Geometry: final body of the model. Coordinates: model frame, mm. A direction names the side the tool comes from. Give positions to 0.01 mm unless a question says otherwise; leave off trailing zeros. Write each loop counter-clockwise with the first axis right and the second up, starting at its lowest first coordinate (ties: lowest second). Pieces come first, ordered by that corner, then holes. Notation, with made-up numbers: M 4,58.25 L 48,58.25 A4 ccw 48,62.25 Z; hole C 33,24.5 d7. An arc over 180 degrees is marked long. Use one line per item in the form item = value. Start each with the question number.
Item 1: Section query A-A on z = -1.5. Return loops of the section in (x, y), then the cut area to 3 significant figures.
Item 2: Access query for faces 1 (the flat face through (-7.9, 2, 5)), 2 (the flat face through (-12.5, 0, 2)), 3 (the flat face through (10.25, -4, 11)), 4 (the flat face through (14.25, -4, 9)). Directions: +Z, -Z, +X, -X, +Y, -Y. A direction counts if a zero-diameter tool reaches every point of the face in a straight line with its end or side. Return the directions, or none.
Item 3: Material intervals for line 1 along Z through (x, y) = (21.3, 0); line 2 along Z through (x, y) = (12.25, -4.2); line 3 along X through (y, z) = (-3, 2), sorted ascending. Write a range as from..to.
Item 4: Contact query for flat-ended pins moving along their axis: P1, Ø2, axis at y = 3, z = 3, coming from the -X side; P2, Ø1.3, axis at y = -3.5, z = 11, coming from the +X side; P3, Ø6, axis at x = 16.5, z = 8.5, coming from the +Y side. Output: stop coordinate, or through.
Item 5: Section query B-B on x = 17.5. Return loops of the section in (y, z).
Item 6: Section query D-D on y = -1.75. Return loops of the section in (x, z), then the cut area to 3 significant figures.
Item 7: Section query C-C on z = 14.9. Return loops of the section in (x, y), then the cut area to 3 significant figures.
Item 8: Pull-direction query (X, two-part tool) for faces 5 (the flat face through (-12, -4, 16.9)), 6 (the cylindrical face through (-16.576, -0.383, 0.71)), 7 (the flat face through (-14.25, -4, 9)); classes: released by +X, released by -X, zero draft, split by the parting line, or undercut.
from build123d import *

# Parameters (mm, degrees)
F1_DEPTH = 4.5
F2_R     = 0.75
F3_DEPTH = 43.801
F4_R     = 1
F5_DEPTH = 1.2
F6_R     = 1
F6_W     = 15.8
F6_H     = 4.5
F7_DEPTH = 11.401


with BuildPart() as f1:
    # F0 (on Front) → F1 (new body, symmetric)
    with BuildSketch(Plane.XZ):
        Polygon((12.5, 4), (12.5, 0), (20.5, 0), (20.5, -6), (21.9, -6), (21.9, 1.4), (13.9, 1.4), (13.9, 5.4), (-13.9, 5.4), (-13.9, 1.4), (-21.9, 1.4), (-21.9, -6), (-20.5, -6), (-20.5, 0), (-12.5, 0), (-12.5, 4), align=None)
    extrude(amount=F1_DEPTH, both=True)

    # F2 (on face) → F3 (cut, through all)
    with BuildSketch(Plane.YZ.offset(21.9)):
        with Locations((0, -3.5)):
            Circle(F2_R)
    extrude(amount=-F3_DEPTH, mode=Mode.SUBTRACT)

    # F4 (on face) → F5 (join)
    with BuildSketch(Plane.XZ.offset(4.5)):
        Polygon((14.25, 16.9), (10.25, 16.9), (10.25, 5.4), (13.9, 5.4), (13.9, 1.4), (14.25, 1.4), align=None)
        with Locations((12.25, 14.9)):
            Circle(F4_R, mode=Mode.SUBTRACT)
        Polygon((-10.25, 16.9), (-14.25, 16.9), (-14.25, 1.4), (-13.9, 1.4), (-13.9, 5.4), (-10.25, 5.4), align=None)
        with Locations((-12.25, 14.9)):
            Circle(F4_R, mode=Mode.SUBTRACT)
    extrude(amount=-F5_DEPTH)

    # F6 (on face) → F7 (cut, through all)
    with BuildSketch(Plane.XY.offset(5.4)):
        with Locations((-17.5, 0)):
            Circle(F6_R)
        with Locations((17.5, 0)):
            Circle(F6_R)
        with Locations((0, 2.25)):
            Rectangle(F6_W, F6_H)
    extrude(amount=-F7_DEPTH, mode=Mode.SUBTRACT)


solid = f1.part
Answer sheet:
q1.outline = M -21.9,-4.5 L -20.5,-4.5 L -20.5,4.5 L -21.9,4.5 Z; M 20.5,-4.5 L 21.9,-4.5 L 21.9,4.5 L 20.5,4.5 Z
q1.area = 25.2 mm2
q2.face_1 = +Z, -Z, +Y
q2.face_2 = -Z, +Y, -Y
q2.face_3 = +Z, +Y, -Y
q2.face_4 = +Z, +X, +Y, -Y
q3.line_1 = -6..-4.25, -2.75..1.4
q3.line_2 = 4..13.9, 15.9..16.9
q3.line_3 = -13.9..-12.5, 12.5..13.9
q4.P1 = -13.9
q4.P2 = 14.25
q4.P3 = -3.3
q5.outline = M -4.5,0 L -1,0 L -1,1.4 L -4.5,1.4 Z; M 1,0 L 4.5,0 L 4.5,1.4 L 1,1.4 Z
q6.outline = M -21.9,-6 L -20.5,-6 L -20.5,0 L -12.5,0 L -12.5,4 L 12.5,4 L 12.5,0 L 20.5,0 L 20.5,-6 L 21.9,-6 L 21.9,1.4 L 13.9,1.4 L 13.9,5.4 L -13.9,5.4 L -13.9,1.4 L -21.9,1.4 Z
q6.area = 89.3 mm2
q7.outline = M -14.25,-4.5 L -13.25,-4.5 L -13.25,-3.3 L -14.25,-3.3 Z; M -11.25,-4.5 L -10.25,-4.5 L -10.25,-3.3 L -11.25,-3.3 Z; M 10.25,-4.5 L 11.25,-4.5 L 11.25,-3.3 L 10.25,-3.3 Z; M 13.25,-4.5 L 14.25,-4.5 L 14.25,-3.3 L 13.25,-3.3 Z
q7.area = 4.80 mm2
q8.face_5 = zero draft
q8.face_6 = undercut
q8.face_7 = released by -X
